Could you check a few things on this model? Use its own coordinates, in mm. A direction names the side the tool comes from. Round coordinates to 2 decimals unless told otherwise and drop trailing zeros. Loops run counter-clockwise (first coordinate to the right, second up) from the corner with the lowest first, then second, coordinate; pieces in that order, holes last. Notation, with made-up numbers: (-20, -21) -> (5, -21) arc R17 ccw to (5, 3) -> close; hole circle Ø3 at (24.5, 88.5). An arc over 180 degrees is marked (long way). One line per item, written item: value.
```python
from build123d import *

# Parameters (mm, degrees)
SKETCH_2_R      = 1.912823122
EXTRUDE_1_DEPTH = 15


with BuildPart() as part:
    # Эскиз2 → Бобышка-Вытянуть1 (new body)
    with BuildSketch(Plane.XY):
        with BuildLine():
            ThreePointArc((44.312740246, 4.037123861), (49.962876139, 4.312740246), (49.687259754, 9.962876139))
            Line((49.687259754, 9.962876139), (46.841765339, 12.543673399))
            ThreePointArc((46.841765339, 12.543673399), (42.631280931, 45.388335386), (9.532754169, 46.382078879))
            Line((9.532754169, 46.382078879), (6.687259754, 48.962876139))
            ThreePointArc((6.687259754, 48.962876139), (1.037123861, 48.687259754), (1.312740246, 43.037123861))
            Line((1.312740246, 43.037123861), (4.158234661, 40.456326601))
            ThreePointArc((4.158234661, 40.456326601), (1.061659056, 33.78131114), (0, 26.5))
            Line((0, 26.5), (0, 0))
            Line((0, 0), (20, 0))
            Line((20, 0), (20, 1.600200804))
            ThreePointArc((20, 1.600200804), (31.30389422, 1.669276855), (41.467245831, 6.617921121))
            Line((41.467245831, 6.617921121), (44.312740246, 4.037123861))
        make_face()
        with Locations((47, 7)):
            Circle(SKETCH_2_R, mode=Mode.SUBTRACT)
        with Locations((4, 46)):
            Circle(SKETCH_2_R, mode=Mode.SUBTRACT)
    extrude(amount=EXTRUDE_1_DEPTH)


solid = part.part
```
Item 1: If we section it at D-D on x = 13: List the corners of the cut face in (y, z) for me.
Output:
outline: (0, 0) -> (48.73, 0) -> (48.73, 15) -> (0, 15) -> close
Item 2: If we section it at C-C on y = 20: List the corners of the cut face in (x, z) for me, plus the area to 3 significant figures.
Output:
outline: (0, 0) -> (50.16, 0) -> (50.16, 15) -> (0, 15) -> close
area: 752 mm²
Item 3: For faces 1 (the face through (48.28, 11.24, 7.4)), 2 (the face through (20, 1, 7)), 3 (the face through (8.13, 47.654, 7.395)), 4 (the face through (1.09, 33.88, 7.4)), which set-ups out of +Z, -Z, +X, -X, +Y, -Y let a thin tool reach every point of the face, with its end or its side?
Output:
face 1: +Z, -Z, +X
face 2: +Z, -Z, -Y
face 3: +Z, -Z, +Y
face 4: +Z, -Z, -X
Item 4: If we mould it in two halves opening along X, with no side actions, what happens to faces 5 (the face through (31.148, 1.633, 7.395)), 6 (the face through (1.097, 48.752, 7.395)), 7 (the face through (10, 0, 7)), 8 (the face through (2.72, 41.76, 7.4))? For each: released by +X, released by -X, zero draft, split by the parting line, or undercut.
Output:
face 5: undercut
face 6: undercut
face 7: zero draft
face 8: released by -X
Item 5: I need wall thicknesses on line 1 (Y direction, x = 47, z = 7.75); line 2 (Y direction, x = 48, z = 1.5); line 3 (Y direction, x = 26, z = 8.75). Which ranges of each line are inside material? Lowest first, please. Write a range as from..to.
Output:
line 1: y = 3..5.09, 8.91..12.4, 12.79..40.21
line 2: y = 3.13..5.37, 8.63..11.49, 14.5..38.5
line 3: y = 1..52
Item 6: If we section it at A-A on z = 12.25: List the corners of the cut face in (x, y) for me, plus the area to 3 significant figures.
Output:
outline: (0, 0) -> (20, 0) -> (20, 1.6) arc R25.5 ccw to (41.47, 6.62) -> (44.31, 4.04) arc R4 ccw to (49.69, 9.96) -> (46.84, 12.54) arc R25.5 ccw to (9.53, 46.38) -> (6.69, 48.96) arc R4 ccw to (1.31, 43.04) -> (4.16, 40.46) arc R25.5 ccw to (0, 26.5) -> close; hole circle Ø3.83 at (4, 46); hole circle Ø3.83 at (47, 7)
area: 2,290 mm²
Item 7: If we section it at B-B on x = 46: List the corners of the cut face in (y, z) for me.
Output:
outline: (3.13, 0) -> (5.37, 0) -> (5.37, 15) -> (3.13, 15) -> close; (8.63, 0) -> (41.67, 0) -> (41.67, 15) -> (8.63, 15) -> close
Item 8: Will these pins go through, and if not, where does the flat tip stop? pin 1 Ø4 at (y, z) = (33, 2) entering from -X; pin 2 Ø3 at (x, y) = (47, 7) entering from +Z; pin 3 Ø2 at (x, z) = (24.5, 11) entering from -Y; pin 4 Ø4.5 at (x, y) = (4, 46) entering from +Z.
Output:
pin 1: stops at x = 0.4
pin 2: passes through
pin 3: stops at y = 1
pin 4: stops at z = 15
